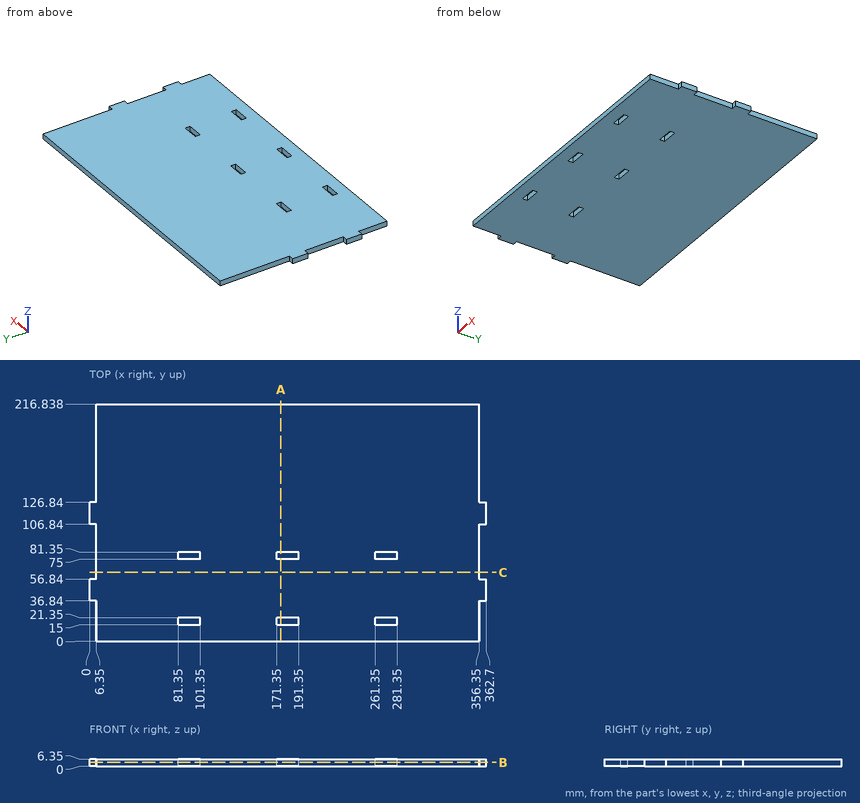
For this review, use the dimensioned drawing (mm, ordinates from the lowest corner) and the shaded views. Round coordinates to 2 decimals unless told otherwise and drop trailing zeros. Write each loop counter-clockwise with the first axis right and the second up, starting at its lowest first coordinate (ties: lowest second). Pieces come first, ordered by that corner, then holes. Notation, with made-up numbers: M 4,27 L 47,27 A18 ccw 47,62 Z; hole C 21.5,17 d3. An arc over 180 degrees is marked long. Write item = value, one per line. Start each with the question number.
(1) For line 1 along Y through (x, z) = (100.5, 2); line 2 along X through (y, z) = (170, 3), list the stretches that pass through material, from the lowest coordinate up.
(2) We need section A-A (x = 175). Give the boundary of the cut face in (y, z).
(3) Clearance check with flat-ended pins moving along their axes: pin 1 Ø3 at (x, z) = (4, 2.5) entering from +Y; pin 2 Ø3 at (y, z) = (31.5, 3) entering from +X; pin 3 Ø3 at (y, z) = (18, 3) entering from -X. State where each tip first meets the part, or that it passes through.
(4) We need section C-C (y = 63). Give the boundary of the cut face in (x, z).
(5) We need section B-B (z = 3.5). Give the number of separate pieces and of enclosed holes in the cut face, then the cut area to 3 significant figures.
Results found:
q1.line_1 = 0 to 15, 21.35 to 75, 81.35 to 216.84
q1.line_2 = 6.35 to 356.35
q2.outline = M 0,0 L 15,0 L 15,6.35 L 0,6.35 Z; M 21.35,0 L 75,0 L 75,6.35 L 21.35,6.35 Z; M 81.35,0 L 216.84,0 L 216.84,6.35 L 81.35,6.35 Z
q3.pin_1 = 126.84
q3.pin_2 = 356.35
q3.pin_3 = 6.35
q4.outline = M 6.35,0 L 356.35,0 L 356.35,6.35 L 6.35,6.35 Z
q5.separate_pieces = 1
q5.enclosed_holes = 6
q5.area = 75,600 mm²
